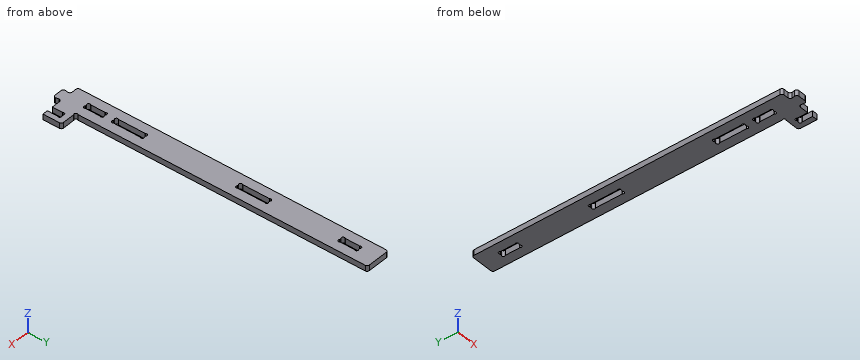
from build123d import *

# Parameters (mm, degrees)
BOSS_EXTRUDE1_DEPTH = 18
CUT_EXTRUDE1_DEPTH  = 19
CUT_EXTRUDE2_DEPTH  = 19
CUT_EXTRUDE3_DEPTH  = 19
LPATTERN1_COUNT     = 2
LPATTERN1_PITCH     = 400
FILLET1_R           = 7


with BuildPart() as part:
    # Sketch1 → Boss-Extrude1 (new body)
    with BuildSketch(Plane.XY):
        with BuildLine():
            Line((0, 0), (30, 0))
            Line((30, 0), (26, -25))
            Line((26, -25), (66, -25))
            Line((66, -25), (62, 0))
            Line((62, 0), (134, 0))
            Line((134, 0), (134, 60))
            Line((134, 60), (87.987761491, 60))
            ThreePointArc((87.987761491, 60), (87.206612206, 59.874827529), (86.503685629, 59.511844635))
            ThreePointArc((86.503685629, 59.511844635), (80, 60), (79.511844635, 66.503685629))
            ThreePointArc((79.511844635, 66.503685629), (79.874827529, 67.206612206), (80, 67.987761491))
            Line((80, 67.987761491), (80, 1000))
            Line((80, 1000), (0, 1000))
            Line((0, 1000), (0, 0))
        make_face()
    extrude(amount=BOSS_EXTRUDE1_DEPTH)

    # Sketch2 → Cut-Extrude1 (cut, through all)
    with BuildSketch(Plane.XY):
        with BuildLine():
            Line((49.5, 642.748771852), (49.5, 557.251228148))
            ThreePointArc((49.5, 557.251228148), (49.599672829, 556.660561143), (49.88765279, 556.135309084))
            ThreePointArc((49.88765279, 556.135309084), (49.5, 549.5), (42.864690916, 549.11234721))
            ThreePointArc((42.864690916, 549.11234721), (42.339438857, 549.400327171), (41.748771852, 549.5))
            Line((41.748771852, 549.5), (38.251228148, 549.5))
            ThreePointArc((38.251228148, 549.5), (37.660561143, 549.400327171), (37.135309084, 549.11234721))
            ThreePointArc((37.135309084, 549.11234721), (30.5, 549.5), (30.11234721, 556.135309084))
            ThreePointArc((30.11234721, 556.135309084), (30.400327171, 556.660561143), (30.5, 557.251228148))
            Line((30.5, 557.251228148), (30.5, 642.748771852))
            ThreePointArc((30.5, 642.748771852), (30.400327171, 643.339438857), (30.11234721, 643.864690916))
            ThreePointArc((30.11234721, 643.864690916), (30.5, 650.5), (37.135309084, 650.88765279))
            ThreePointArc((37.135309084, 650.88765279), (37.660561143, 650.599672829), (38.251228148, 650.5))
            Line((38.251228148, 650.5), (41.748771852, 650.5))
            ThreePointArc((41.748771852, 650.5), (42.339438857, 650.599672829), (42.864690916, 650.88765279))
            ThreePointArc((42.864690916, 650.88765279), (49.5, 650.5), (49.88765279, 643.864690916))
            ThreePointArc((49.88765279, 643.864690916), (49.599672829, 643.339438857), (49.5, 642.748771852))
        make_face()
    cut_extrude1 = extrude(amount=CUT_EXTRUDE1_DEPTH, mode=Mode.SUBTRACT)

    # Sketch3 → Cut-Extrude2 (cut, through all)
    with BuildSketch(Plane.XY):
        with BuildLine():
            Line((98, 0), (117, 0))
            Line((117, 0), (117, 32.748771852))
            ThreePointArc((117, 32.748771852), (117.099672829, 33.339438857), (117.38765279, 33.864690916))
            ThreePointArc((117.38765279, 33.864690916), (117, 40.5), (110.364690916, 40.88765279))
            ThreePointArc((110.364690916, 40.88765279), (109.839438857, 40.599672829), (109.248771852, 40.5))
            Line((109.248771852, 40.5), (105.751228148, 40.5))
            ThreePointArc((105.751228148, 40.5), (105.160561143, 40.599672829), (104.635309084, 40.88765279))
            ThreePointArc((104.635309084, 40.88765279), (98, 40.5), (97.61234721, 33.864690916))
            ThreePointArc((97.61234721, 33.864690916), (97.900327171, 33.339438857), (98, 32.748771852))
            Line((98, 32.748771852), (98, 0))
        make_face()
    extrude(amount=CUT_EXTRUDE2_DEPTH, mode=Mode.SUBTRACT)

    # Sketch4 → Cut-Extrude3 (cut, through all)
    with BuildSketch(Plane.XY):
        with BuildLine():
            Line((49.5, 113.248771852), (49.5, 67.751228148))
            ThreePointArc((49.5, 67.751228148), (49.599672829, 67.160561143), (49.88765279, 66.635309084))
            ThreePointArc((49.88765279, 66.635309084), (49.5, 60), (42.864690916, 59.61234721))
            ThreePointArc((42.864690916, 59.61234721), (42.339438857, 59.900327171), (41.748771852, 60))
            Line((41.748771852, 60), (38.251228148, 60))
            ThreePointArc((38.251228148, 60), (37.660561143, 59.900327171), (37.135309084, 59.61234721))
            ThreePointArc((37.135309084, 59.61234721), (30.5, 60), (30.11234721, 66.635309084))
            ThreePointArc((30.11234721, 66.635309084), (30.400327171, 67.160561143), (30.5, 67.751228148))
            Line((30.5, 67.751228148), (30.5, 113.248771852))
            ThreePointArc((30.5, 113.248771852), (30.400327171, 113.839438857), (30.11234721, 114.364690916))
            ThreePointArc((30.11234721, 114.364690916), (30.5, 121), (37.135309084, 121.38765279))
            ThreePointArc((37.135309084, 121.38765279), (37.660561143, 121.099672829), (38.251228148, 121))
            Line((38.251228148, 121), (41.748771852, 121))
            ThreePointArc((41.748771852, 121), (42.339438857, 121.099672829), (42.864690916, 121.38765279))
            ThreePointArc((42.864690916, 121.38765279), (49.5, 121), (49.88765279, 114.364690916))
            ThreePointArc((49.88765279, 114.364690916), (49.599672829, 113.839438857), (49.5, 113.248771852))
        make_face()
        with BuildLine():
            Line((38.251228148, 879.5), (41.748771852, 879.5))
            ThreePointArc((41.748771852, 879.5), (42.339438857, 879.400327171), (42.864690916, 879.11234721))
            ThreePointArc((42.864690916, 879.11234721), (49.5, 879.5), (49.88765279, 886.135309084))
            ThreePointArc((49.88765279, 886.135309084), (49.599672829, 886.660561143), (49.5, 887.251228148))
            Line((49.5, 887.251228148), (49.5, 932.748771852))
            ThreePointArc((49.5, 932.748771852), (49.599672829, 933.339438857), (49.88765279, 933.864690916))
            ThreePointArc((49.88765279, 933.864690916), (49.5, 940.5), (42.864690916, 940.88765279))
            ThreePointArc((42.864690916, 940.88765279), (42.339438857, 940.599672829), (41.748771852, 940.5))
            Line((41.748771852, 940.5), (38.251228148, 940.5))
            ThreePointArc((38.251228148, 940.5), (37.660561143, 940.599672829), (37.135309084, 940.88765279))
            ThreePointArc((37.135309084, 940.88765279), (30.5, 940.5), (30.11234721, 933.864690916))
            ThreePointArc((30.11234721, 933.864690916), (30.400327171, 933.339438857), (30.5, 932.748771852))
            Line((30.5, 932.748771852), (30.5, 887.251228148))
            ThreePointArc((30.5, 887.251228148), (30.400327171, 886.660561143), (30.11234721, 886.135309084))
            ThreePointArc((30.11234721, 886.135309084), (30.5, 879.5), (37.135309084, 879.11234721))
            ThreePointArc((37.135309084, 879.11234721), (37.660561143, 879.400327171), (38.251228148, 879.5))
        make_face()
    extrude(amount=CUT_EXTRUDE3_DEPTH, mode=Mode.SUBTRACT)

    # LPattern1: Cut-Extrude1 ×2
    with Locations(*[(0, -i * LPATTERN1_PITCH, 0) for i in range(1, LPATTERN1_COUNT)]):
        add(cut_extrude1, mode=Mode.SUBTRACT)

    # Fillet1
    fillet1_edges = [part.edges().sort_by_distance(p)[0] for p in [
        (0, 0, 9),
        (0, 1000, 9),
        (80, 1000, 9),
        (134, 60, 9),
        (62, 0, 9),
        (66, -25, 9),
        (26, -25, 9),
        (30, 0, 9),
    ]]
    fillet(fillet1_edges, radius=FILLET1_R)


solid = part.part
Geometry: final body of the model. Coordinates: model frame, mm. Coordinates: 2 decimals unless noted, no trailing zeros. Order: outer loops, then holes, each group sorted by start corner. A loop starts at its lowest first (then second) coordinate and runs counter-clockwise, first axis right, second up. Notation, with made-up numbers: M -24,51.5 L 2,51.5 A26 ccw 2,88.5 Z; hole C 0,29 d7. An arc over 180 degrees is marked long. One line per question, with ' | ' between items. Start each with the question number.
Item 1: Cut plane B-B, the plane z = 3.5. Count the separate pieces of the cut face and the enclosed holes in it, then the cut area to 3 significant figures.
Item 2: Ray query, probe 1 along X at (y, z) = (894, 11); probe 2 along X at (y, z) = (553, 3.75); probe 3 along Y at (x, z) = (94.5, 14). Return the intervals inside material, ascending. Write a range as [from, to].
Item 3: Cut plane C-C, the plane y = 524. Return the cut outline in (x, z).
Item 4: Pin query (flat end, axial travel): pin 1 Ø5.5 at (y, z) = (221.5, 10.5) entering from +X; pin 2 Ø2 at (x, z) = (85.5, 14.5) entering from -Y. Return the tip coordinate at first contact, or that it passes through.
Item 5: Cut plane A-A, the plane y = 199. Return the cut outline in (x, z).
A:
1) separate pieces: 1 | enclosed holes: 4 | area: 76,900 mm2
2) probe 1: x = [0, 30.5], [49.5, 80] | probe 2: x = [0, 29.04], [50.96, 80] | probe 3: y = [0, 60]
3) outline: M 0,0 L 80,0 L 80,18 L 0,18 Z
4) pin 1: stops at x = 80 | pin 2: stops at y = 0
5) outline: M 0,0 L 30.5,0 L 30.5,18 L 0,18 Z; M 49.5,0 L 80,0 L 80,18 L 49.5,18 Z
